from build123d import *

# Parameters (mm, degrees)
F0_W      = 60
F0_H      = 55
F1_DEPTH  = 6
F2_W      = 54
F2_H      = 49
F3_DEPTH  = 1
F4_W      = 48
F4_H      = 43
F5_DEPTH  = 25
F6_R      = 3
F7_DEPTH  = 6
F8_DEPTH  = 54
F9_R      = 1
F10_DEPTH = 25
F11_R     = 3
F12_R     = 1


with BuildPart() as f1:
    # F0 (on Top) → F1 (new body)
    with BuildSketch(Plane.XY):
        with Locations((12.012976855, 12.1693141837)):
            Rectangle(F0_W, F0_H)
    extrude(amount=F1_DEPTH)

    # F2 (on face) → F3 (cut)
    with BuildSketch(Plane.XY.offset(6)):
        with Locations((12.012976855, 12.1693141837)):
            Rectangle(F2_W, F2_H)
    extrude(amount=-F3_DEPTH, mode=Mode.SUBTRACT)

    # F4 (on face) → F5 (cut)
    with BuildSketch(Plane.XY.offset(5)):
        with Locations((12.012976855, 12.1693141837)):
            Rectangle(F4_W, F4_H)
    extrude(amount=-F5_DEPTH, mode=Mode.SUBTRACT)

    # F6 (on face) → F7 (join, through all)
    with BuildSketch(Plane.XY.offset(6)):
        with Locations((-10.487023145, 32.1693141837)):
            Circle(F6_R)
        with Locations((34.512976855, 32.1693141837)):
            Circle(F6_R)
        with Locations((34.512976855, -7.8306858163)):
            Circle(F6_R)
        with Locations((-10.487023145, -7.8306858163)):
            Circle(F6_R)
    extrude(amount=-F7_DEPTH)

    # F8 (cut, through all): a face of the model
    f8_faces = [f1.faces().sort_by_distance(p)[0] for p in [
        (39.012976855, 12.1693141837, 5.5),
    ]]
    extrude(f8_faces, amount=F8_DEPTH, mode=Mode.SUBTRACT)

    # F9 (on face) → F10 (cut)
    with BuildSketch(Plane.XY.offset(6)):
        with Locations((-10.487023145, -7.8306858163)):
            Circle(F9_R)
        with Locations((34.512976855, -7.8306858163)):
            Circle(F9_R)
        with Locations((34.512976855, 32.1693141837)):
            Circle(F9_R)
        with Locations((-10.487023145, 32.1693141837)):
            Circle(F9_R)
    extrude(amount=-F10_DEPTH, mode=Mode.SUBTRACT)

    # F11
    f11_edges = [f1.edges().sort_by_distance(p)[0] for p in [
        (-7.888947, 33.669314, 2.5),
        (-11.987023, 29.571238, 2.5),
        (36.012977, 29.571238, 2.5),
        (31.914901, 33.669314, 2.5),
        (36.012977, -5.23261, 2.5),
        (31.914901, -9.330686, 2.5),
        (-11.987023, -5.23261, 2.5),
        (-7.888947, -9.330686, 2.5),
    ]]
    fillet(f11_edges, radius=F11_R)

    # F12
    f12_edges = [f1.edges().sort_by_distance(p)[0] for p in [
        (-17.987023, -15.330686, 3),
        (-17.987023, 39.669314, 3),
        (42.012977, 39.669314, 3),
        (42.012977, -15.330686, 3),
        (39.012977, 36.669314, 5.5),
        (-14.987023, 36.669314, 5.5),
        (-14.987023, -12.330686, 5.5),
        (39.012977, -12.330686, 5.5),
    ]]
    fillet(f12_edges, radius=F12_R)


solid = f1.part
The listing builds one solid part. Answer for the finished solid, in the listing's coordinates (mm). A direction names the side the tool comes from. Give positions to 0.01 mm unless a question says otherwise; leave off trailing zeros. Order: outer loops, then holes, each group sorted by start corner. A loop starts at its lowest first (then second) coordinate and runs counter-clockwise, first axis right, second up. Notation, with made-up numbers: (51.25, -33) - (91.25, -33) arc R34 ccw to (91.25, -2) - close; hole circle Ø1 at (18, 46.5). An arc over 180 degrees is marked (long way). Use one line per item in the form item = value.
1) The mould has two halves that part along X. Classify faces 1 (the flat face through (36.013, 12, 3)), 2 (the flat face through (12, 37, 0)), 3 (the flat face through (-17.987, 12, 3)): released by +X, released by -X, zero draft, split by the parting line, or undercut.
Verdict:
face_1 = undercut
face_2 = zero draft
face_3 = released by -X
2) For faces 4 (the flat face through (12, 39.669, 3)), 5 (the flat face through (12, 33.669, 3)), 6 (the flat face through (16, -10, 5)), determine the directions among +Z, -Z, +X, -X, +Y, -Y from which every point of the face is accessible in a straight line to the end or side of a thin tool.
Verdict:
face_4 = +Z, -Z, +X, -X, +Y
face_5 = +Z, -Z
face_6 = +Z
3) Each of these flat-tipped pins is pushed along its axis until it touches: pin 1 (12 mm diameter, centred on x = 13.5, y = 27, fed in from +Z); pin 2 (3 mm diameter, centred on x = 34.51, y = -7.83, fed in from +Z). Where does it stop, or does it pass through?
Verdict:
pin_1 = through
pin_2 = 5
4) Find section C-C on z = 2.55. Determine the outline of the cut face in (x, y), and give its area (3 significant figures).
Verdict:
outline = (-17.99, -14.33) arc R1 ccw to (-16.99, -15.33) - (41.01, -15.33) arc R1 ccw to (42.01, -14.33) - (42.01, 38.67) arc R1 ccw to (41.01, 39.67) - (-16.99, 39.67) arc R1 ccw to (-17.99, 38.67) - close; hole (-11.99, -2.02) arc R3 ccw to (-9.74, -4.93) arc R3 cw to (-7.58, -7.08) arc R3 ccw to (-4.68, -9.33) - (28.7, -9.33) arc R3 ccw to (31.61, -7.08) arc R3 cw to (33.76, -4.93) arc R3 ccw to (36.01, -2.02) - (36.01, 26.36) arc R3 ccw to (33.76, 29.26) arc R3 cw to (31.61, 31.42) arc R3 ccw to (28.7, 33.67) - (-4.68, 33.67) arc R3 ccw to (-7.58, 31.42) arc R3 cw to (-9.74, 29.26) arc R3 ccw to (-11.99, 26.36) - close; hole circle Ø2 at (-10.49, -7.83); hole circle Ø2 at (-10.49, 32.17); hole circle Ø2 at (34.51, -7.83); hole circle Ø2 at (34.51, 32.17)
area = 1,310 mm^2
5) Consider probe 1 along Y at (x, z) = (12, 1.25); probe 2 along X at (y, z) = (23.5, 5.05); probe 3 along X at (y, z) = (-1.5, 2.3). Determine where each line is inside the solid, lowest interval first. Write a range as [from, to].
Verdict:
probe_1 = [-15.33, -9.33], [33.67, 39.67]
probe_2 = [-17.99, -14.99], [39.01, 42.01]
probe_3 = [-17.99, -11.99], [36.01, 42.01]
6) Find section A-A on y = 19. Determine the outline of the cut face in (x, z).
Verdict:
outline = (-17.99, 0) - (-11.99, 0) - (-11.99, 5) - (-14.99, 5) - (-14.99, 6) - (-17.99, 6) - close; (36.01, 0) - (42.01, 0) - (42.01, 6) - (39.01, 6) - (39.01, 5) - (36.01, 5) - close
7) Find section B-B on x = 4.5. Determine the outline of the cut face in (y, z), and give its area (3 significant figures).
Verdict:
outline = (-15.33, 0) - (-9.33, 0) - (-9.33, 5) - (-12.33, 5) - (-12.33, 6) - (-15.33, 6) - close; (33.67, 0) - (39.67, 0) - (39.67, 6) - (36.67, 6) - (36.67, 5) - (33.67, 5) - close
area = 66.0 mm^2
